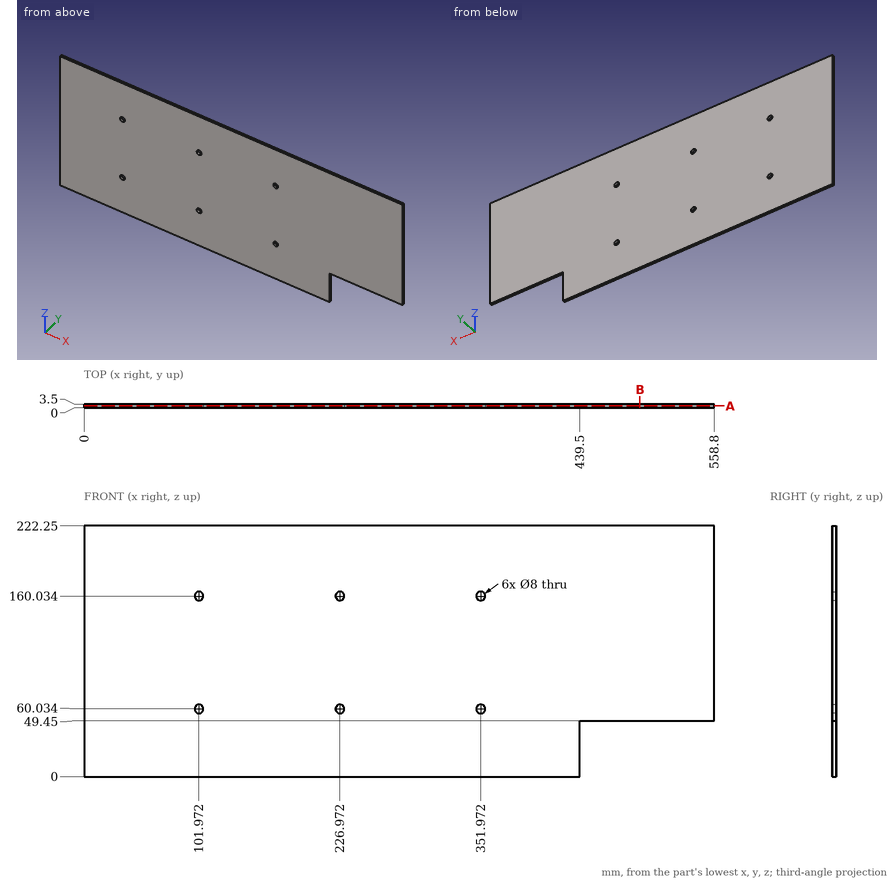
The figure shows three views and two pictorial views of one solid part (mm, origin at its lowest corner). Answer the questions. Give positions to 0.01 mm unless a question says otherwise; leave off trailing zeros. Loops run counter-clockwise (first coordinate to the right, second up) from the corner with the lowest first, then second, coordinate; pieces in that order, holes last. Notation, with made-up numbers: (40.25, 51.25) -> (61.25, 51.25) arc R30 cw to (61.25, 83.25) -> close; hole circle Ø4 at (9.25, 15.5). An arc over 180 degrees is marked (long way). Use a Markdown table: item, result. Add a question column.
1. Section A-A on y = 1.85 is taken. Determine the outline of the cut face in (x, z), and give its area (3 significant figures).
2. Find the intervals of material crossed by probe 1 along X at (y, z) = (1.7, 39.5); probe 2 along Z at (x, y) = (468, 0.95), in increasing order.
3. Section B-B on x = 493 is taken. Determine the outline of the cut face in (y, z), and give its area (3 significant figures).
4. Flat-ended cylindrical pins translate along their axes: pin 1 Ø1 at (y, z) = (1, 23) entering from +X; pin 2 Ø1 at (x, y) = (487.5, 2.5) entering from -Z; pin 3 Ø7 at (x, z) = (101.97, 160.03) entering from -Y. Find the tip coordinate at first contact, or state that the pin passes through.
Results below:
| question | item | result |
|---|---|---|
| 1 | outline | (0, 0) -> (439.5, 0) -> (439.5, 49.45) -> (558.8, 49.45) -> (558.8, 222.25) -> (0, 222.25) -> close; hole circle Ø8 at (101.97, 60.03); hole circle Ø8 at (101.97, 160.03); hole circle Ø8 at (226.97, 60.03); hole circle Ø8 at (226.97, 160.03); hole circle Ø8 at (351.97, 60.03); hole circle Ø8 at (351.97, 160.03) |
| 1 | area | 118,000 mm^2 |
| 2 | probe 1 | x = 0 to 439.5 |
| 2 | probe 2 | z = 49.45 to 222.25 |
| 3 | outline | (0, 49.45) -> (3.5, 49.45) -> (3.5, 222.25) -> (0, 222.25) -> close |
| 3 | area | 605 mm^2 |
| 4 | pin 1 | stops at x = 439.5 |
| 4 | pin 2 | stops at z = 49.45 |
| 4 | pin 3 | passes through |
